Input: part model. Units: mm. Frame: model coordinates. A direction names the side the tool comes from. Coordinates: 2 decimals unless noted, no trailing zeros. Write each loop counter-clockwise with the first axis right and the second up, starting at its lowest first coordinate (ties: lowest second). Pieces come first, ordered by that corner, then holes.
1) Pin query (flat end, axial travel): pin 1 Ø8 at (y, z) = (-14, -6) entering from -X; pin 2 Ø2 at (x, y) = (-1.5, 5) entering from +Z; pin 3 Ø2 at (y, z) = (-2, -2.5) entering from +X; pin 4 Ø3 at (x, y) = (-1.5, 7) entering from -Z (3 decimals). Return the tip coordinate at first contact, or that it passes through.
2) Set-up query: faces 1 (the cylindrical face through (2.66, 4.24, -4.18)), 2 (the cylindrical face through (-6.269, 0.74, 4.807)), 3 (the cylindrical face through (1.29, -9.962, -2.024)), 4 (the cylindrical face through (-1.4, -6.83, -0.06)). Return all of +Z, -Z, +X, -X, +Y, -Y with unobstructed straight access to the full face (end or side cutting, diameter ignored); none if empty.
3) Section query A-A (y = 6). Output: boundary loops of the cut face in (x, z) (3 decimals).
4) Section query C-C (x = 6.75). Output: boundary loops of the cut face in (y, z).
5) Draft query along Y for faces 5 (the flat face through (1.1, -4.5, 1.1)), 6 (the flat face through (0, -9.1, 2)), 7 (the conical face through (0.963, -14.57, -0.303)), 8 (the flat face through (-2, 14.15, 0)). Return one class per face: pulls with the +Y half, pulls with the -Y half, needs draft (parallel to the pull), parting line crosses it, or undercut.
6) Section query B-B (z = 6.5). Output: boundary loops of the cut face in (x, y).
7) Line query: L1, parallel to Z at x = 0, y = 10.25 (3 decimals); L2, parallel to Z at x = 0, y = -3.25; L3, parallel to X at y = -10.75, z = 0. Output: solid intervals per line, ascending.
from build123d import *

# Parameters (mm, degrees)
FILLET1_R = 0.75
FILLET2_R = 0.1


with BuildPart() as part:
    # Sketch1 → Revolve1 (revolve)
    with BuildSketch(Plane.XY):
        Polygon((1.5, 14.15), (2.5, 14.15), (3.475, 13.15), (3.475, 12.65), (2.75, 11.95), (2.75, 11.05), (3.475, 10.35), (3.475, 7.15), (4.955, 7.15), (4.955, 1.5), (7.9, 1.5), (7.9, 0), (5.85, 0), (5.85, -4.5), (1.4, -4.5), (1.4, -9.1), (2.4, -9.1), (2.4, -10.8), (0.15, -16.9), (0.15, 0), (1.5, 0), align=None)
    revolve(axis=Axis((0, 0, 0), (0, 1, 0)))

    # Fillet1
    fillet1_edges = [part.edges().sort_by_distance(p)[0] for p in [
        (-5.85, -4.5, 0),
    ]]
    fillet(fillet1_edges, radius=FILLET1_R)

    # Fillet2
    fillet2_edges = [part.edges().sort_by_distance(p)[0] for p in [
        (-4.955, 7.15, 0),
        (-3.475, 10.35, 0),
    ]]
    fillet(fillet2_edges, radius=FILLET2_R)


solid = part.part
Answer:
1. pin 1: passes through
1. pin 2: stops at z = 4.93
1. pin 3: stops at x = 5.65
1. pin 4: stops at z = -4.955
2. face 1: +Y
2. face 2: +Y, -Y
2. face 3: -Y
2. face 4: none
3. outline: circle Ø9.91 at (0, 0); hole circle Ø3 at (0, 0)
4. outline: (0, -4.1) - (1.5, -4.1) - (1.5, 4.1) - (0, 4.1) - close
5. face 5: undercut
5. face 6: undercut
5. face 7: pulls with the -Y half
5. face 8: pulls with the +Y half
6. outline: (-4.49, 0) - (4.49, 0) - (4.49, 1.5) - (-4.49, 1.5) - close
7. L1: z = -3.475 to -1.5, 1.5 to 3.475
7. L2: z = -5.85 to -0.15, 0.15 to 5.85
7. L3: x = -2.4 to -0.15, 0.15 to 2.4
